Geometry check sheet. Reference: the model listing, model coordinates, mm. A direction names the side the tool comes from. Coordinates: 2 decimals unless noted, no trailing zeros. Write each loop counter-clockwise with the first axis right and the second up, starting at its lowest first coordinate (ties: lowest second). Pieces come first, ordered by that corner, then holes. Notation, with made-up numbers: M 3,63.5 L 34,63.5 A25 ccw 34,101.5 Z; hole C 78,28 d8. An arc over 180 degrees is marked long. Write each question's results on one line, items separated by ' | '.
```python
from build123d import *

# Parameters (mm, degrees)
SKETCH1_R            = 75
SKETCH1_R_2          = 70
BOSS_EXTRUDE1_DEPTH  = 22.5
SKETCH2_R            = 75
BOSS_EXTRUDE2_DEPTH  = 5
SKETCH4_R            = 1.5
CUT_EXTRUDE2_DEPTH   = 5
SKETCH5_R            = 2.5
CUT_EXTRUDE3_DEPTH   = 10
LPATTERN1_COUNT      = 2
LPATTERN1_PITCH      = 20
LPATTERN1_COUNT_DIR2 = 2
LPATTERN1_PITCH_DIR2 = 20
SKETCH6_R            = 2.5
CUT_EXTRUDE4_DEPTH   = 10
SKETCH8_R            = 7.5
BOSS_EXTRUDE3_DEPTH  = 7
CUT_EXTRUDE5_DEPTH   = 7


with BuildPart() as part:
    # Sketch1 → Boss-Extrude1 (new body)
    with BuildSketch(Plane(origin=(0, 0, 0), x_dir=(1, 0, 0), z_dir=(0, 1, 0))):
        Circle(SKETCH1_R)
        Circle(SKETCH1_R_2, mode=Mode.SUBTRACT)
    extrude(amount=BOSS_EXTRUDE1_DEPTH)

    # Sketch2 → Boss-Extrude2 (add)
    with BuildSketch(Plane(origin=(0, 22.5, 0), x_dir=(1, 0, 0), z_dir=(0, 1, 0))):
        Circle(SKETCH2_R)
    extrude(amount=BOSS_EXTRUDE2_DEPTH)

    # Sketch4 → Cut-Extrude2 (cut)
    with BuildSketch(Plane(origin=(0, 27.5, 0), x_dir=(1, 0, 0), z_dir=(0, 1, 0))):
        Circle(SKETCH4_R)
    extrude(amount=-CUT_EXTRUDE2_DEPTH, mode=Mode.SUBTRACT)

    # Sketch5 → Cut-Extrude3 (cut)
    with BuildSketch(Plane(origin=(0, 27.5, 0), x_dir=(1, 0, 0), z_dir=(0, 1, 0))):
        with Locations((-10, 10)):
            Circle(SKETCH5_R)
    cut_extrude3 = extrude(amount=-CUT_EXTRUDE3_DEPTH, mode=Mode.SUBTRACT)

    # LPattern1: Cut-Extrude3 2 × 2
    with Locations(*[(j * LPATTERN1_PITCH_DIR2, 0, i * LPATTERN1_PITCH) for i in range(LPATTERN1_COUNT) for j in range(LPATTERN1_COUNT_DIR2) if (i, j) != (0, 0)]):
        add(cut_extrude3, mode=Mode.SUBTRACT)

    # Sketch6 → Cut-Extrude4 (cut)
    with BuildSketch(Plane(origin=(0, 27.5, 0), x_dir=(1, 0, 0), z_dir=(0, 1, 0))):
        with Locations((-25.844790679, 33.64590309)):
            Circle(SKETCH6_R)
        with Locations((33.64590309, 25.844790679)):
            Circle(SKETCH6_R)
        with Locations((-33.64590309, -25.844790679)):
            Circle(SKETCH6_R)
        with Locations((25.844790679, -33.64590309)):
            Circle(SKETCH6_R)
    extrude(amount=-CUT_EXTRUDE4_DEPTH, mode=Mode.SUBTRACT)

    # Sketch8 → Boss-Extrude3 (add)
    with BuildSketch(Plane.XZ.offset(-22.5)):
        with Locations((-33.64590309, 25.844790679)):
            Circle(SKETCH8_R)
        with Locations((25.844790679, 33.64590309)):
            Circle(SKETCH8_R)
        with Locations((33.64590309, -25.844790679)):
            Circle(SKETCH8_R)
        with Locations((-25.844790679, -33.64590309)):
            Circle(SKETCH8_R)
    extrude(amount=BOSS_EXTRUDE3_DEPTH)

    # Sketch7 → Cut-Extrude5 (cut)
    with BuildSketch(Plane.XZ.offset(-22.5)):
        Polygon((-31.336502014, 29.844790679), (-35.955304167, 29.844790679), (-38.264705244, 25.844790679), (-35.955304167, 21.844790679), (-31.336502014, 21.844790679), (-29.027100937, 25.844790679), align=None)
        Polygon((28.154191756, 37.64590309), (23.535389602, 37.64590309), (21.225988525, 33.64590309), (23.535389602, 29.64590309), (28.154191756, 29.64590309), (30.463592832, 33.64590309), align=None)
        Polygon((35.955304167, -21.844790679), (31.336502014, -21.844790679), (29.027100937, -25.844790679), (31.336502014, -29.844790679), (35.955304167, -29.844790679), (38.264705244, -25.844790679), align=None)
        Polygon((-23.535389602, -29.64590309), (-28.154191756, -29.64590309), (-30.463592832, -33.64590309), (-28.154191756, -37.64590309), (-23.535389602, -37.64590309), (-21.225988525, -33.64590309), align=None)
    extrude(amount=CUT_EXTRUDE5_DEPTH, mode=Mode.SUBTRACT)


solid = part.part
```
Q1. Depth check by flat-ended pin: P1, Ø8, axis at x = 47, y = 4.5, coming from the +Z side; P2, Ø5, axis at x = 34, y = 18, coming from the +Z side; P3, Ø4, axis at y = 11, z = -20, coming from the -X side. Enter the tip coordinate at first touch or a pass-through.
Geometry check:
P1: stops at z = 61.45 | P2: stops at z = 68.06 | P3: stops at x = -72.81
Q2. Sectioned sample at C-C on z = -10. Record the cut outline in (x, y).
Geometry check:
outline: M -74.33,0 L -69.28,0 L -69.28,22.5 L -12.5,22.5 L -12.5,27.5 L -74.33,27.5 Z; M -7.5,22.5 L 7.5,22.5 L 7.5,27.5 L -7.5,27.5 Z; M 12.5,22.5 L 69.28,22.5 L 69.28,0 L 74.33,0 L 74.33,27.5 L 12.5,27.5 Z
Q3. Sectioned sample at D-D on z = 44.5. Record the cut outline in (x, y), and give its area (3 significant figures).
Geometry check:
outline: M -60.37,0 L -54.03,0 L -54.03,22.5 L 54.03,22.5 L 54.03,0 L 60.37,0 L 60.37,27.5 L -60.37,27.5 Z | area: 889 mm2
Q4. Sectioned sample at B-B on x = -10. Record the cut outline in (y, z), and give its area (3 significant figures).
Geometry check:
outline: M 0,-74.33 L 27.5,-74.33 L 27.5,-12.5 L 22.5,-12.5 L 22.5,-69.28 L 0,-69.28 Z; M 0,69.28 L 22.5,69.28 L 22.5,12.5 L 27.5,12.5 L 27.5,74.33 L 0,74.33 Z; M 22.5,-7.5 L 27.5,-7.5 L 27.5,7.5 L 22.5,7.5 Z | area: 920 mm2
Q5. Access from +Z, -Z, +X, -X, +Y, -Y to the whole of each face (thin tool, end or side, straight path). Record for faces 4 (the cylindrical face through (9.46, 25.04, 12.44)), 5 (the flat face through (-29.325, 19.049, -35.618)).
Geometry check:
face 4: +Y, -Y | face 5: -Y
Q6. Sectioned sample at A-A on y = 24.25. Give the number of separate pieces and of enclosed holes in the cut face, and give its area (3 significant figures).
Geometry check:
separate pieces: 1 | enclosed holes: 9 | area: 17,500 mm2
Q7. Mould release check, pull along Z, two halves, no side actions. Record for faces 1 (the flat face through (-30.198, 19.049, 23.817)), 2 (the flat face through (50, 0, 50)), 3 (the cylindrical face through (-9.764, 13.558, -74.362)): pulls with the +Z half, pulls with the -Z half, needs draft (parallel to the pull), parting line crosses it, or undercut.
Geometry check:
face 1: undercut | face 2: needs draft | face 3: parting line crosses it
Q8. Scan lines: probe 1 along Z at (x, y) = (10, 24.75); probe 2 along X at (y, z) = (9.5, 0); probe 3 along Y at (x, z) = (30, 16). Record each from-to range of solid material in increasing order.
Geometry check:
probe 1: z = -74.33 to -12.5, -7.5 to 7.5, 12.5 to 74.33 | probe 2: x = -75 to -70, 70 to 75 | probe 3: y = 22.5 to 27.5
